Job drawing, mm, ordinate dimensions from the low corner. One solid piece. A direction names the side the tool comes from. Coordinates: 2 decimals unless noted, no trailing zeros. Write each loop counter-clockwise with the first axis right and the second up, starting at its lowest first coordinate (ties: lowest second). Pieces come first, ordered by that corner, then holes.
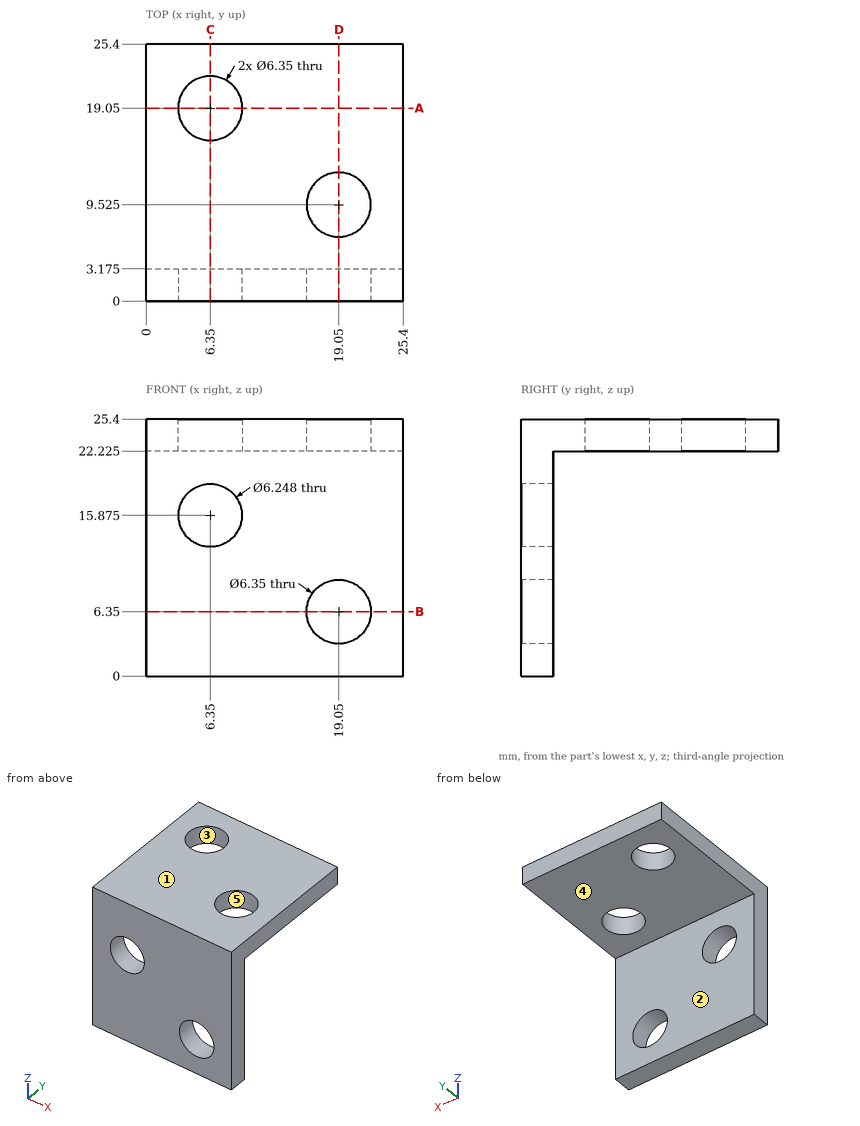
1. Saw through at A-A on y = 19.05. List the corners of the cut face in (x, z) (3 decimals).
Computed values:
outline: (0, 22.225) - (3.175, 22.225) - (3.175, 25.4) - (0, 25.4) - close; (9.525, 22.225) - (25.4, 22.225) - (25.4, 25.4) - (9.525, 25.4) - close
2. Saw through at C-C on x = 6.35. List the corners of the cut face in (y, z) (3 decimals).
Computed values:
outline: (0, 0) - (3.175, 0) - (3.175, 12.751) - (0, 12.751) - close; (0, 18.999) - (3.175, 18.999) - (3.175, 22.225) - (15.875, 22.225) - (15.875, 25.4) - (0, 25.4) - close; (22.225, 22.225) - (25.4, 22.225) - (25.4, 25.4) - (22.225, 25.4) - close
3. Saw through at D-D on x = 19.05. List the corners of the cut face in (y, z) (3 decimals), plus the area to 3 significant figures.
Computed values:
outline: (0, 0) - (3.175, 0) - (3.175, 3.175) - (0, 3.175) - close; (0, 9.525) - (3.175, 9.525) - (3.175, 22.225) - (6.35, 22.225) - (6.35, 25.4) - (0, 25.4) - close; (12.7, 22.225) - (25.4, 22.225) - (25.4, 25.4) - (12.7, 25.4) - close
area: 111 mm2
4. 3-axis set-ups, long thin cutter, end or side, ignore diameter. For the marked faces 1 and 2: which of +Z, -Z, +X, -X, +Y, -Y reach the whole face in a straight line?
Computed values:
face 1: +Z, +X, -X, +Y, -Y
face 2: -Z, +X, -X, +Y
5. Mould opens along X. For the marked faces 3, 4 and 5 say: +X half, -X half, draft (parallel to the pull), parting line (faces both ways), or undercut.
Computed values:
face 3: undercut
face 4: draft
face 5: undercut
6. Probe line 1 along Y through (x, z) = (6.35, 23) (3 decimals); line 2 along Y through (x, z) = (19.05, 22.95); line 3 along Z through (x, y) = (19.05, 1.5) (3 decimals). List the from-to ranges inside material, lowest first.
Computed values:
line 1: y = 0 to 15.875, 22.225 to 25.4
line 2: y = 0 to 6.35, 12.7 to 25.4
line 3: z = 0 to 3.175, 9.525 to 25.4
7. Flat gauge pins, fed straight in: pin 1 (12 mm diameter, centred on x = 16, y = 19.5, fed in from -Z) (3 decimals); pin 2 (7 mm diameter, centred on x = 6.35, z = 15.875, fed in from +Y) (3 decimals). Where does each tip first touch, or does it go through?
Computed values:
pin 1: stops at z = 22.225
pin 2: stops at y = 3.175
8. Saw through at B-B on z = 6.35. List the corners of the cut face in (x, y) (3 decimals).
Computed values:
outline: (0, 0) - (15.875, 0) - (15.875, 3.175) - (0, 3.175) - close; (22.225, 0) - (25.4, 0) - (25.4, 3.175) - (22.225, 3.175) - close
